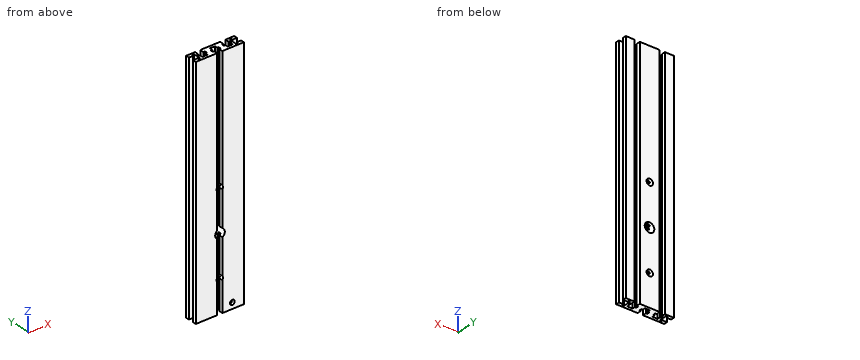
```python
from build123d import *

# Parameters (mm, degrees)
EXTRUDE_1_DEPTH         = 300
HOLE_WIZARD_12_0_12_1_D = 12
HOLE_WIZARD_8_0_8_1_D   = 8
HOLE_WIZARD_6_0_6_1_D   = 6


with BuildPart() as part:
    # 草图1 → 凸台-拉伸1 (new body)
    with BuildSketch(Plane.XY):
        Polygon((0, 0), (26.75, 0), (26.75, 4.796419132), (24.926505169, 4.796419132), (24.926505169, 8.023402897), (26.75, 8.023402897), (26.75, 11.5), (30, 11.5), (33.25, 11.5), (33.25, 8.023402897), (35.073494831, 8.023402897), (35.073494831, 4.796419132), (33.25, 4.796419132), (33.25, 0), (60, 0), (60, 4.25), (54.613325713, 4.25), (54.613325713, 2.4), (52.2, 2.4), (52.2, 12.6), (54.613325713, 12.6), (54.613325713, 10.75), (60, 10.75), (60, 15), (48.947608979, 15), (48.947608979, 10.003848618), (50.733802833, 10.003848618), (50.733802833, 7.094693738), (48.947608979, 7.094693738), (48.947608979, 3.5), (42.447608979, 3.5), (42.447608979, 7.094693738), (40.533802833, 7.094693738), (40.533802833, 10.003848618), (42.447608979, 10.003848618), (42.447608979, 15), (30, 15), (17.552391021, 15), (17.552391021, 10.003848618), (19.466197167, 10.003848618), (19.466197167, 7.094693738), (17.552391021, 7.094693738), (17.552391021, 3.5), (11.052391021, 3.5), (11.052391021, 7.094693738), (9.266197167, 7.094693738), (9.266197167, 10.003848618), (11.052391021, 10.003848618), (11.052391021, 15), (0, 15), (0, 10.75), (5.386674287, 10.75), (5.386674287, 12.6), (7.8, 12.6), (7.8, 2.4), (5.386674287, 2.4), (5.386674287, 4.25), (0, 4.25), align=None)
    extrude(amount=EXTRUDE_1_DEPTH)

    # Ø12.0 (12) 直径孔1 (through all)
    with Locations(Plane(origin=(0, 15, 0), x_dir=(1, 0, 0), z_dir=(0, 1, 0))):
        with Locations((30.31545922, -92)):
            Hole(HOLE_WIZARD_12_0_12_1_D / 2)

    # Ø8.0 (8) 直径孔1 (through all)
    with Locations(Plane(origin=(0, 15, 0), x_dir=(1, 0, 0), z_dir=(0, 1, 0))):
        with Locations((30, -40), (30, -144)):
            Hole(HOLE_WIZARD_8_0_8_1_D / 2)

    # Ø6.0 (6) 直径孔1 (through all)
    with Locations(Plane(origin=(0, 3.5, 0), x_dir=(1, 0, 0), z_dir=(0, 1, 0))):
        with Locations((45.697608979, -7.5)):
            Hole(HOLE_WIZARD_6_0_6_1_D / 2)


solid = part.part
```
Check sheet for the modelled part. Datum: model origin and axes. Units: mm. Coordinates: 2 decimals unless noted, no trailing zeros. Write each loop counter-clockwise with the first axis right and the second up, starting at its lowest first coordinate (ties: lowest second). Pieces come first, ordered by that corner, then holes. Notation, with made-up numbers: M -4,78 L 18,78 A11 cw 18,87 Z; hole C -19.75,47.5 d7. An arc over 180 degrees is marked long. Write item = value, one per line. Start each with the question number.
1. Sectioned sample at A-A (x = 30). Record the cut outline in (y, z).
2. Go/stop test with flat-tipped pins: pin 1 (1.5 mm diameter, centred on y = 7, z = 258, fed in from -X); pin 2 (1 mm diameter, centred on y = 10, z = 219, fed in from +X); pin 3 (2 mm diameter, centred on x = 31.5, y = 6.5, fed in from -Z). Record where each tip stops, or that it passes through.
3. Thickness scan on probe 1 along X at (y, z) = (9, 92); probe 2 along X at (y, z) = (12.5, 164); probe 3 along X at (y, z) = (13.5, 56). Record the ranges inside material, lowest first.
The answers:
q1.outline = M 11.5,0 L 15,0 L 15,36 L 11.5,36 Z; M 11.5,44 L 15,44 L 15,86.01 L 11.5,86.01 Z; M 11.5,97.99 L 15,97.99 L 15,140 L 11.5,140 Z; M 11.5,148 L 15,148 L 15,300 L 11.5,300 Z
q2.pin_1 = 7.8
q2.pin_2 = 52.2
q2.pin_3 = through
q3.probe_1 = 7.8 to 9.27, 19.47 to 24.32, 36.32 to 40.53, 50.73 to 52.2
q3.probe_2 = 0 to 5.39, 7.8 to 11.05, 17.55 to 42.45, 48.95 to 52.2, 54.61 to 60
q3.probe_3 = 0 to 11.05, 17.55 to 42.45, 48.95 to 60
